```python
from build123d import *

# Parameters (mm, degrees)
SKETCH069_W     = 68
SKETCH069_H     = 36
SKETCH069_W_2   = 3.04
SKETCH069_H_2   = 13.335
PAD048_DEPTH    = 1
SKETCH070_W     = 68
SKETCH070_H     = 36
SKETCH070_W_2   = 66
SKETCH070_H_2   = 34
PAD049_DEPTH    = 13
SKETCH073_R     = 1.5
POCKET013_DEPTH = 1.001


with BuildPart() as part:
    # Sketch069 → Pad048 (new body)
    with BuildSketch(Plane.XY):
        Rectangle(SKETCH069_W, SKETCH069_H)
        with Locations((-24.94, 4.5625)):
            Rectangle(SKETCH069_W_2, SKETCH069_H_2, mode=Mode.SUBTRACT)
    extrude(amount=PAD048_DEPTH)

    # Sketch070 (on Face10 of Pad048) → Pad049 (join)
    with BuildSketch(Plane.XY.offset(1)):
        Rectangle(SKETCH070_W, SKETCH070_H)
        Rectangle(SKETCH070_W_2, SKETCH070_H_2, mode=Mode.SUBTRACT)
    extrude(amount=PAD049_DEPTH)

    # Sketch073 (on Face15 of Pad049) → Pocket013 (cut, through all)
    with BuildSketch(Plane.XY.offset(1)):
        with Locations((-31, 15)):
            Circle(SKETCH073_R)
        with Locations((31, 15)):
            Circle(SKETCH073_R)
        with Locations((31, -15)):
            Circle(SKETCH073_R)
        with Locations((-31, -15)):
            Circle(SKETCH073_R)
    extrude(amount=-POCKET013_DEPTH, mode=Mode.SUBTRACT)


solid = part.part
```
Verification items for the finished model (mm, model axes). A direction names the side the tool comes from. Round coordinates to 2 decimals unless told otherwise and drop trailing zeros. Write each loop counter-clockwise with the first axis right and the second up, starting at its lowest first coordinate (ties: lowest second). Pieces come first, ordered by that corner, then holes. Notation, with made-up numbers: (68, 60.5) - (90, 60.5) arc R21 ccw to (90, 86.5) - close; hole circle Ø6 at (-37.75, -6.5). An arc over 180 degrees is marked (long way). Answer as a JSON object with one key per item and string values. Group by question number.
Q1. Thickness scan on line 1 (Y direction, x = 31, z = 0.3); line 2 (Y direction, x = 30, z = 5.25); line 3 (X direction, y = -15.5, z = 5). Record the ranges inside material, lowest first.
Q2. Section check D-D, the plane y = -15. Enter the section's corners in (x, z), plus the area to 3 significant figures.
Q3. Section check B-B, the plane x = -31. Enter the section's corners in (y, z), plus the area to 3 significant figures.
Q4. Mould release check, pull along Y, two halves, no side actions. Record for faces 3 (the flat face through (33, 0, 7)), 4 (the flat face through (0, 0, 0)), 5 (the flat face through (0, 18, 7)): released by +Y, released by -Y, zero draft, split by the parting line, or undercut.
Q5. Section check A-A, the plane y = 2.5. Enter the section's corners in (x, z), plus the area to 3 significant figures.
Q6. Tool access check on faces 1 (the flat face through (0, 17, 7)), 2 (the cylindrical face through (29.5, 15.07, 0.51)). Record the directions out of +Z, -Z, +X, -X, +Y, -Y that give a thin tool (end or side, any length) a straight path to the whole face; none if there is none.
Q7. Section check C-C, the plane z = 8.5. Enter the section's corners in (x, y), plus the area to 3 significant figures.
Found:
{
 "1": {"line 1": "y = -18 to -16.5, -13.5 to 13.5, 16.5 to 18", "line 2": "y = -18 to -17, 17 to 18", "line 3": "x = -34 to -33, 33 to 34"},
 "2": {"outline": "(-34, 0) - (-32.5, 0) - (-32.5, 1) - (-33, 1) - (-33, 14) - (-34, 14) - close; (-29.5, 0) - (29.5, 0) - (29.5, 1) - (-29.5, 1) - close; (32.5, 0) - (34, 0) - (34, 14) - (33, 14) - (33, 1) - (32.5, 1) - close", "area": "88.0 mm^2"},
 "3": {"outline": "(-18, 0) - (-16.5, 0) - (-16.5, 1) - (-17, 1) - (-17, 14) - (-18, 14) - close; (-13.5, 0) - (13.5, 0) - (13.5, 1) - (-13.5, 1) - close; (16.5, 0) - (18, 0) - (18, 14) - (17, 14) - (17, 1) - (16.5, 1) - close", "area": "56.0 mm^2"},
 "4": {"face 3": "undercut", "face 4": "zero draft", "face 5": "released by +Y"},
 "5": {"outline": "(-34, 0) - (-26.46, 0) - (-26.46, 1) - (-33, 1) - (-33, 14) - (-34, 14) - close; (-23.42, 0) - (34, 0) - (34, 14) - (33, 14) - (33, 1) - (-23.42, 1) - close", "area": "91.0 mm^2"},
 "6": {"face 1": "+Z", "face 2": "+Z, -Z"},
 "7": {"outline": "(-34, -18) - (34, -18) - (34, 18) - (-34, 18) - close; hole (-33, -17) - (33, -17) - (33, 17) - (-33, 17) - close", "area": "204 mm^2"}
}
